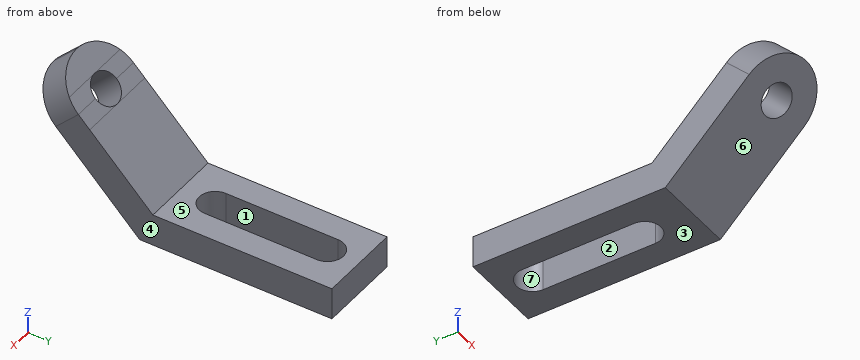
```python
from build123d import *

# Parameters (mm, degrees)
F0_W     = 10
F0_H     = 20
F0_W_2   = 50
F2_DEPTH = 52
F3_R     = 25.99999
F4_D     = 20
F1_W     = 10
F1_H     = 70
F5_DEPTH = 47
F7_D     = 20


# Not quite as in the source:
# - a fillet or chamfer is up to 0.001 mm smaller than in the source, because OpenCascade refuses the exact size


with BuildPart() as f2:
    # F0 (on Right) → F2 (new body)
    with BuildSketch(Plane.YZ):
        with Locations((-5, 10)):
            Rectangle(F0_W, F0_H)
        with Locations((-15, 10)):
            Rectangle(F0_W, F0_H)
        with Locations((-25, 10)):
            Rectangle(F0_W, F0_H)
        with Locations((-55, 10)):
            Rectangle(F0_W_2, F0_H)
        with Locations((-85, 10)):
            Rectangle(F0_W, F0_H)
        with Locations((-95, 10)):
            Rectangle(F0_W, F0_H)
        Polygon((-120, 0), (-100, 0), (-100, 20), (-111.7157287525, 20), (-151.1126983722, 59.3969696197), (-165.2548339959, 45.2548339959), align=None)
        Polygon((-172.3259018078, 52.3259018078), (-165.2548339959, 45.2548339959), (-151.1126983722, 59.3969696197), (-158.1837661841, 66.4680374315), align=None)
        Polygon((-179.3969696197, 59.3969696197), (-172.3259018078, 52.3259018078), (-158.1837661841, 66.4680374315), (-165.2548339959, 73.5391052434), align=None)
        Polygon((-190.7106781187, 70.7106781187), (-179.3969696197, 59.3969696197), (-165.2548339959, 73.5391052434), (-176.5685424949, 84.8528137424), align=None)
    extrude(amount=F2_DEPTH)

    # F3 (radius 26 in the source; OpenCascade refuses exactly that, so slightly less here)
    f3_edges = [f2.edges().sort_by_distance(p)[0] for p in [
        (52, -183.63961, 77.781746),
        (0, -183.63961, 77.781746),
    ]]
    fillet(f3_edges, radius=F3_R)

    # F4 (through all)
    with Locations(Plane(origin=(0, 0, 0), x_dir=(1, 0, 0), z_dir=(0, 0, -1))):
        with Locations((26, 90.0006328523), (26, 20.0006328523)):
            Hole(F4_D / 2)

    # F1 (on Top) → F5 (cut)
    with BuildSketch(Plane.XY):
        with Locations((31, -55.0006328523)):
            Rectangle(F1_W, F1_H)
        with Locations((21, -55.0006328523)):
            Rectangle(F1_W, F1_H)
    extrude(amount=F5_DEPTH, mode=Mode.SUBTRACT)

    # F7 (through all)
    with Locations(Plane(origin=(0, -45.8578643763, -45.8578643763), x_dir=(-1, 0, 0), z_dir=(0, 0.7071067812, 0.7071067812))):
        with Locations((-26, 158.8528137424)):
            Hole(F7_D / 2)


solid = f2.part
```
For this review, take the finished solid that the model builds, in its own axes (mm). Face numbers are marked on the shaded views. A direction names the side the tool comes from. Give positions to 0.01 mm unless a question says otherwise; leave off trailing zeros. Order: outer loops, then holes, each group sorted by start corner. A loop starts at its lowest first (then second) coordinate and runs counter-clockwise, first axis right, second up.
1) Take a section at D-D (x = 7.5). Give the boundary of the cut face in (y, z), then the cut area to 3 significant figures.
2) Take a section at A-A (y = -26). Give the boundary of the cut face in (x, z), then the cut area to 3 significant figures.
3) Take a section at B-B (x = 33). Give the boundary of the cut face in (y, z).
4) Insertion check: pin 1 (2 mm diameter, centred on x = 10, z = 37, fed in from +Y); pin 2 (4 mm diameter, centred on x = 14.5, z = 73.5, fed in from +Y); pin 3 (10 mm diameter, centred on x = 5.5, y = -86.5, fed in from +Z). Each pin has a flat end and moves straight along its axis. Give the tip position at first contact, or say it passes through.
5) Wall thickness on line 1 (X direction, y = -38.5, z = 14); line 2 (Z direction, x = 11.5, y = -106); line 3 (Y direction, x = 34, z = 58): over which ranges is each line inside the solid? List them lowest first.
6) The part is to be moulded in two halves that separate along X. For the marked faces 1, 2, 3 and 4, say which applies: released by +X, released by -X, zero draft, split by the parting line, or undercut.
7) For the marked faces 5, 6 and 7, list the 3-axis set-ups (+Z, -Z, +X, -X, +Y, -Y) from which the entire face can be reached by the end or side of a thin tool; tool diameter is ignored.
8) Take a section at C-C (x = 20). Give the boundary of the cut face in (y, z), then the cut area to 3 significant figures.
Derived:
1. outline: (-185.24, 65.24) - (-120, 0) - (0, 0) - (0, 20) - (-111.72, 20) - (-171.1, 79.39) - close
1. area: 4,080 mm2
2. outline: (0, 0) - (16, 0) - (16, 20) - (0, 20) - close; (36, 0) - (52, 0) - (52, 20) - (36, 20) - close
2. area: 640 mm2
3. outline: (-190.03, 70.03) - (-177.38, 57.38) - (-163.23, 71.52) - (-175.89, 84.17) - close; (-167.28, 47.28) - (-120, 0) - (-97.14, 0) - (-97.14, 20) - (-111.72, 20) - (-153.13, 61.42) - close; (-12.86, 0) - (0, 0) - (0, 20) - (-12.86, 20) - close
4. pin 1: stops at y = -127.72
4. pin 2: stops at y = -163.22
4. pin 3: stops at z = 20
5. line 1: x = 0 to 16, 36 to 52
5. line 2: z = 0 to 20
5. line 3: y = -178 to -175.14, -158.17 to -149.72
6. face 1: undercut
6. face 2: undercut
6. face 3: zero draft
6. face 4: released by +X
7. face 5: +Z, +X, -X, +Y
7. face 6: -Z, +X, -X, -Y
7. face 7: +Z, -Z
8. outline: (-190.21, 70.21) - (-177.98, 57.98) - (-163.84, 72.12) - (-176.07, 84.36) - close; (-166.67, 46.67) - (-120, 0) - (-98, 0) - (-98, 20) - (-111.72, 20) - (-152.53, 60.81) - close; (-12, 0) - (0, 0) - (0, 20) - (-12, 20) - close
8. area: 2,180 mm2
